from build123d import *

# Parameters (mm, degrees)
SKETCH2_R           = 1.4
BOSS_EXTRUDE1_DEPTH = 2.5


with BuildPart() as part:
    # Sketch2 → Boss-Extrude1 (new body)
    with BuildSketch(Plane(origin=(0, 0, 0), x_dir=(1, 0, 0), z_dir=(0, 1, 0))):
        Polygon((-20.1, 55.5), (-20.1, -5.6), (20.1, -5.6), (20.1, 55.5), (14.55, 55.5), (14.55, 0), (-14.55, 0), (-14.55, 55.5), align=None)
        with Locations(Location((-11, -2.8, 0), (0, 0, 270))):
            Circle(SKETCH2_R, mode=Mode.SUBTRACT)
        with Locations(Location((11, -2.8, 0), (0, 0, 90))):
            Circle(SKETCH2_R, mode=Mode.SUBTRACT)
        with Locations(Location((-17.325, 46.5, 0), (0, 0, 270))):
            Circle(SKETCH2_R, mode=Mode.SUBTRACT)
        with Locations(Location((-17.325, 24.5, 0), (0, 0, 270))):
            Circle(SKETCH2_R, mode=Mode.SUBTRACT)
        with Locations(Location((-17.325, 2.5, 0), (0, 0, 270))):
            Circle(SKETCH2_R, mode=Mode.SUBTRACT)
        with Locations(Location((17.325, 46.5, 0), (0, 0, 90))):
            Circle(SKETCH2_R, mode=Mode.SUBTRACT)
        with Locations(Location((17.325, 24.5, 0), (0, 0, 90))):
            Circle(SKETCH2_R, mode=Mode.SUBTRACT)
        with Locations(Location((17.325, 2.5, 0), (0, 0, 90))):
            Circle(SKETCH2_R, mode=Mode.SUBTRACT)
    extrude(amount=BOSS_EXTRUDE1_DEPTH)


solid = part.part
Geometry: final body of the model. Coordinates: model frame, mm. A direction names the side the tool comes from. Round coordinates to 2 decimals unless told otherwise and drop trailing zeros. Loops run counter-clockwise (first coordinate to the right, second up) from the corner with the lowest first, then second, coordinate; pieces in that order, holes last. Notation, with made-up numbers: M -25,14.5 L 22,14.5 A25 cw 22,46.5 Z; hole C 65.25,-32.5 d8. An arc over 180 degrees is marked long. Put each result on its own line as item: value. Start each with the question number.
(1) Section query C-C (x = 11). Return loops of the section in (y, z), then the cut area to 3 significant figures.
(2) Set-up query: faces 4 (the face through (18.692, 1.232, -2.197)), 5 (the face through (0, 1, 0)). Return all of +Z, -Z, +X, -X, +Y, -Y with unobstructed straight access to the full face (end or side cutting, diameter ignored); none if empty.
(3) Section query A-A (z = -6). Return loops of the section in (x, y), then the cut area to 4 significant figures.
(4) Material intervals for line 1 along X through (y, z) = (0.7, -24.5) (3 decimals); line 2 along X through (y, z) = (1.55, 2.8); line 3 along Z through (x, y) = (17.5, 1.3), sorted ascending. Write a range as [from, to].
(5) Contact query for flat-ended pins moving along their axis: pin 1 Ø0.8 at (x, y) = (-4.5, 0.5) entering from -Z; pin 2 Ø1.7 at (x, z) = (-17.325, -2.5) entering from -Y. Output: stop coordinate, or through.
(6) Section query D-D (z = -24.5). Return loops of the section in (x, y) (3 decimals), then the cut area to 4 significant figures.
(7) Section query B-B (z = 2.8). Return loops of the section in (x, y).
(8) Draft query along Z for faces 1 (the face through (17.861, 1.232, -47.793)), 2 (the face through (-15, 2.5, -18)), 3 (the face through (-17, 1, -55.5)). Return one class per face: +Z half, -Z half, draft (parallel to the pull), parting line (faces both ways), or undercut.
Findings below:
1. outline: M 0,0 L 2.5,0 L 2.5,1.4 L 0,1.4 Z; M 0,4.2 L 2.5,4.2 L 2.5,5.6 L 0,5.6 Z
1. area: 7.00 mm2
2. face 4: +Y, -Y
2. face 5: -Z, +Y, -Y
3. outline: M -20.1,0 L -14.55,0 L -14.55,2.5 L -20.1,2.5 Z; M 14.55,0 L 20.1,0 L 20.1,2.5 L 14.55,2.5 Z
3. area: 27.75 mm2
4. line 1: x = [-20.1, -18.725], [-15.925, -14.55], [14.55, 15.925], [18.725, 20.1]
4. line 2: x = [-20.1, -12.4], [-9.6, 9.6], [12.4, 20.1]
4. line 3: z = [-55.5, -47.89], [-45.11, -25.89], [-23.11, -3.89], [-1.11, 5.6]
5. pin 1: stops at z = 0
5. pin 2: passes through
6. outline: M -20.1,0 L -18.725,0 L -18.725,2.5 L -20.1,2.5 Z; M -15.925,0 L -14.55,0 L -14.55,2.5 L -15.925,2.5 Z; M 14.55,0 L 15.925,0 L 15.925,2.5 L 14.55,2.5 Z; M 18.725,0 L 20.1,0 L 20.1,2.5 L 18.725,2.5 Z
6. area: 13.75 mm2
7. outline: M -20.1,0 L -12.4,0 L -12.4,2.5 L -20.1,2.5 Z; M -9.6,0 L 9.6,0 L 9.6,2.5 L -9.6,2.5 Z; M 12.4,0 L 20.1,0 L 20.1,2.5 L 12.4,2.5 Z
8. face 1: undercut
8. face 2: draft
8. face 3: -Z half
